For this review, take the finished solid that the model builds, in its own axes (mm). A direction names the side the tool comes from. Give positions to 0.01 mm unless a question says otherwise; leave off trailing zeros. Write each loop counter-clockwise with the first axis right and the second up, starting at its lowest first coordinate (ties: lowest second). Pieces come first, ordered by that corner, then holes.
1) We need section B-B on z = 52. Give the boundary of the cut face in (x, y).
2) Machinability: for faces 4 (the face through (-142.28, -119.03, 31.3)), 5 (the face through (23.456, 1.907, -9.392)), 6 (the face through (-142.08, 119.23, 31.3)), which of the approach directions +Z, -Z, +X, -X, +Y, -Y give a long, thin tool a straight path to every point of the face, cutting with its end or side? Answer none if there is none.
3) Wall thickness on line 1 along Y through (x, z) = (59.5, 13.5); line 2 along Z through (x, y) = (-38, 10); line 3 along X through (y, z) = (47.5, 18): over which ranges is each line inside the solid? List them lowest first.
4) We need section C-C on y = 0. Give the boundary of the cut face in (x, z).
5) Draft analysis for pull direction Z (two halves, no side actions). For faces 1 (the face through (142.43, 142.23, 2.38)), 2 (the face through (-22.44, -3.86, -9.39)), 3 (the face through (0, -28, -38.1)), state which applies: pulls with the +Z half, pulls with the -Z half, needs draft (parallel to the pull), parting line crosses it, or undercut.
6) For P1, Ø16, axis at x = 1, z = 32, coming from the -Y side; P2, Ø1.5, axis at y = -109, z = 27.5, coming from the +X side; P3, Ø21, axis at x = 6.5, z = -32, coming from the -Y side, all flat-tipped, find the tip position at first contact; note any pin that passes through.
7) We need section D-D on x = 43.5. Give the boundary of the cut face in (y, z), and give its area (3 significant figures).
8) We need section A-A on x = 5. Give the boundary of the cut face in (y, z), and give its area (3 significant figures).
from build123d import *

# Parameters (mm, degrees)
F1_DEPTH = 4.826
F2_R     = 6.35
F3_DEPTH = 19.05
F5_W     = 50.8
F5_H     = 85.09
F6_DEPTH = 19.05
F8_DEPTH = 53.70068


with BuildPart() as f1:
    # F0 (on Top) → F1 (new body)
    with BuildSketch(Plane.XY):
        with BuildLine():
            ThreePointArc((146.05, 133.35), (142.330256, 142.330256), (133.35, 146.05))
            Line((133.35, 146.05), (-133.35, 146.05))
            ThreePointArc((-133.35, 146.05), (-142.330256, 142.330256), (-146.05, 133.35))
            Line((-146.05, 133.35), (-146.05, -133.35))
            ThreePointArc((-146.05, -133.35), (-142.330256, -142.330256), (-133.35, -146.05))
            Line((-133.35, -146.05), (133.35, -146.05))
            ThreePointArc((133.35, -146.05), (142.330256, -142.330256), (146.05, -133.35))
            Line((146.05, -133.35), (146.05, 133.35))
        make_face()
    extrude(amount=F1_DEPTH)

    # F2 (on Top) → F3 (join)
    with BuildSketch(Plane.XY):
        with Locations((-17.399, -57.15)):
            Circle(F2_R)
        with Locations((17.399, -57.15)):
            Circle(F2_R)
        with Locations((17.399, 0)):
            Circle(F2_R)
        with Locations((-17.399, 0)):
            Circle(F2_R)
    extrude(amount=-F3_DEPTH)

    # F5 (on offset) → F6 (join)
    with BuildSketch(Plane.XY.offset(-19.05)):
        with Locations((0, -28.575)):
            Rectangle(F5_W, F5_H)
    extrude(amount=-F6_DEPTH)

    # F7 (on face) → F8 (join)
    with BuildSketch(Plane.XY.offset(4.826)):
        with BuildLine():
            Line((-133.20014, -122.84964), (133.20014, -122.84964))
            ThreePointArc((133.20014, -122.84964), (142.180396, -119.129896), (145.90014, -110.14964))
            Line((145.90014, -110.14964), (145.90014, 110.14964))
            ThreePointArc((145.90014, 110.14964), (142.180396, 119.129896), (133.20014, 122.84964))
            Line((133.20014, 122.84964), (-133.20014, 122.84964))
            ThreePointArc((-133.20014, 122.84964), (-142.180396, 119.129896), (-145.90014, 110.14964))
            Line((-145.90014, 110.14964), (-145.90014, -110.14964))
            ThreePointArc((-145.90014, -110.14964), (-142.180396, -119.129896), (-133.20014, -122.84964))
        make_face()
    extrude(amount=F8_DEPTH)


solid = f1.part
Results list:
1. outline: (-145.9, -110.15) arc R12.7 ccw to (-133.2, -122.85) - (133.2, -122.85) arc R12.7 ccw to (145.9, -110.15) - (145.9, 110.15) arc R12.7 ccw to (133.2, 122.85) - (-133.2, 122.85) arc R12.7 ccw to (-145.9, 110.15) - close
2. face 4: +Z, -X, -Y
2. face 5: none
2. face 6: +Z, -X, +Y
3. line 1: y = -122.85 to 122.85
3. line 2: z = 0 to 58.53
3. line 3: x = -145.9 to 145.9
4. outline: (-146.05, 0) - (-23.75, 0) - (-23.75, -19.05) - (-25.4, -19.05) - (-25.4, -38.1) - (25.4, -38.1) - (25.4, -19.05) - (23.75, -19.05) - (23.75, 0) - (146.05, 0) - (146.05, 4.83) - (145.9, 4.83) - (145.9, 58.53) - (-145.9, 58.53) - (-145.9, 4.83) - (-146.05, 4.83) - close; hole (-11.05, -19.05) - (11.05, -19.05) - (11.05, 0) - (-11.05, 0) - close
5. face 1: needs draft
5. face 2: undercut
5. face 3: pulls with the -Z half
6. P1: stops at y = -122.85
6. P2: stops at x = 145.9
6. P3: stops at y = -71.12
7. outline: (-146.05, 0) - (146.05, 0) - (146.05, 4.83) - (122.85, 4.83) - (122.85, 58.53) - (-122.85, 58.53) - (-122.85, 4.83) - (-146.05, 4.83) - close
7. area: 14,600 mm2
8. outline: (-146.05, 0) - (146.05, 0) - (146.05, 4.83) - (122.85, 4.83) - (122.85, 58.53) - (-122.85, 58.53) - (-122.85, 4.83) - (-146.05, 4.83) - close; (-71.12, -38.1) - (13.97, -38.1) - (13.97, -19.05) - (-71.12, -19.05) - close
8. area: 16,200 mm2
